from build123d import *

# Parameters (mm, degrees)
CUT_EXTRUDE_1_REACH              = 10
HOLE_WIZARD_M41_AT_2_COUNT       = 2
HOLE_WIZARD_M41_AT_2_PITCH       = 24.04163056
HOLE_WIZARD_M41_AT_3_COUNT       = 2
HOLE_WIZARD_M41_AT_3_PITCH       = 34
HOLE_WIZARD_M41_AT_4_COUNT       = 2
HOLE_WIZARD_M41_AT_4_PITCH       = 24.04163056
HOLE_WIZARD_8_2_8_2_1_AT_2_COUNT = 2
HOLE_WIZARD_8_2_8_2_1_AT_2_PITCH = 29.69848481
HOLE_WIZARD_8_2_8_2_1_AT_3_COUNT = 2
HOLE_WIZARD_8_2_8_2_1_AT_3_PITCH = 42
HOLE_WIZARD_8_2_8_2_1_AT_4_COUNT = 2
HOLE_WIZARD_8_2_8_2_1_AT_4_PITCH = 29.69848481


with BuildPart() as part:
    # Эскиз1 → Повернуть1 (revolve)
    with BuildSketch(Plane.XY):
        with BuildLine():
            Line((7.5, 11), (0.5, 11))
            Line((0.5, 11), (0, 11.5))
            Line((0, 11.5), (0, 25.5))
            Line((0, 25.5), (0.5, 26))
            Line((0.5, 26), (5.5, 26))
            Line((5.5, 26), (6, 25.5))
            Line((6, 25.5), (6, 13.35))
            ThreePointArc((6, 13.35), (6.117157288, 13.067157288), (6.4, 12.95))
            Line((6.4, 12.95), (7.5, 12.95))
            Line((7.5, 12.95), (8, 12.45))
            Line((8, 12.45), (8, 11.5))
            Line((8, 11.5), (7.5, 11))
        make_face()
    revolve(axis=Axis((0, 0, 0), (1, 0, 0)))

    # Эскиз2 → Вырез-Вытянуть1 (cut, up to next)
    with BuildSketch(Plane.ZY, mode=Mode.PRIVATE) as cut_extrude_1_sk1:
        with BuildLine():
            Line((-15.329709717, 21), (15.329709717, 21))
            ThreePointArc((15.329709717, 21), (0, 26), (-15.329709717, 21))
        make_face()
    cut_extrude_1_tool1 = extrude(cut_extrude_1_sk1.sketch, amount=-CUT_EXTRUDE_1_REACH, mode=Mode.PRIVATE) & part.part
    add(cut_extrude_1_tool1.solids().sort_by_distance((0, 23.017458, 0))[0], mode=Mode.SUBTRACT)
    # Эскиз2 → Вырез-Вытянуть1 (cut, up to next)
    with BuildSketch(Plane.ZY, mode=Mode.PRIVATE) as cut_extrude_1_sk2:
        with BuildLine():
            Line((21, 15.329709717), (21, -15.329709717))
            ThreePointArc((21, -15.329709717), (26, 0), (21, 15.329709717))
        make_face()
    cut_extrude_1_tool2 = extrude(cut_extrude_1_sk2.sketch, amount=-CUT_EXTRUDE_1_REACH, mode=Mode.PRIVATE) & part.part
    add(cut_extrude_1_tool2.solids().sort_by_distance((0, 0, 23.017458))[0], mode=Mode.SUBTRACT)
    # Эскиз2 → Вырез-Вытянуть1 (cut, up to next)
    with BuildSketch(Plane.ZY, mode=Mode.PRIVATE) as cut_extrude_1_sk3:
        with BuildLine():
            Line((15.329709717, -21), (-15.329709717, -21))
            ThreePointArc((-15.329709717, -21), (0, -26), (15.329709717, -21))
        make_face()
    cut_extrude_1_tool3 = extrude(cut_extrude_1_sk3.sketch, amount=-CUT_EXTRUDE_1_REACH, mode=Mode.PRIVATE) & part.part
    add(cut_extrude_1_tool3.solids().sort_by_distance((0, -23.017458, 0))[0], mode=Mode.SUBTRACT)
    # Эскиз2 → Вырез-Вытянуть1 (cut, up to next)
    with BuildSketch(Plane.ZY, mode=Mode.PRIVATE) as cut_extrude_1_sk4:
        with BuildLine():
            Line((-21, -15.329709717), (-21, 15.329709717))
            ThreePointArc((-21, 15.329709717), (-26, 0), (-21, -15.329709717))
        make_face()
    cut_extrude_1_tool4 = extrude(cut_extrude_1_sk4.sketch, amount=-CUT_EXTRUDE_1_REACH, mode=Mode.PRIVATE) & part.part
    add(cut_extrude_1_tool4.solids().sort_by_distance((0, 0, -23.017458))[0], mode=Mode.SUBTRACT)

    # Эскиз4 → Цековка для винта с внутренним шестигранником M41 (revolve, cut)
    with BuildSketch(Plane(origin=(0, 15.974774553, 5.814342437), x_dir=(0, 0, 1), z_dir=(0, 1, 0))):
        Polygon((0, 0), (0, 6), (2.4, 6), (2.25, 5.85), (2.25, 4.2), (3.7, 4.2), (3.7, 0.15), (3.85, 0), align=None)
    hole_wizard_m41 = revolve(axis=Axis((-6.35, 15.974774553, 5.814342437), (1, 0, 0)), mode=Mode.SUBTRACT)

    # Цековка для винта с внутренним шестигранником M41 at 2: Цековка для винта с внутренним шестигранником M41 ×2
    with Locations(*[Vector(0, -0.422618262, -0.906307787) * (i * HOLE_WIZARD_M41_AT_2_PITCH) for i in range(1, HOLE_WIZARD_M41_AT_2_COUNT)]):
        add(hole_wizard_m41, mode=Mode.SUBTRACT)

    # Цековка для винта с внутренним шестигранником M41 at 3: Цековка для винта с внутренним шестигранником M41 ×2
    with Locations(*[Vector(0, -0.939692621, -0.342020143) * (i * HOLE_WIZARD_M41_AT_3_PITCH) for i in range(1, HOLE_WIZARD_M41_AT_3_COUNT)]):
        add(hole_wizard_m41, mode=Mode.SUBTRACT)

    # Цековка для винта с внутренним шестигранником M41 at 4: Цековка для винта с внутренним шестигранником M41 ×2
    with Locations(*[Vector(0, -0.906307787, 0.422618262) * (i * HOLE_WIZARD_M41_AT_4_PITCH) for i in range(1, HOLE_WIZARD_M41_AT_4_COUNT)]):
        add(hole_wizard_m41, mode=Mode.SUBTRACT)

    # Эскиз6 → Диаметр отверстия Ø8.2 (8.2)1 (revolve, cut)
    with BuildSketch(Plane(origin=(0, 14.849242405, -14.849242405), x_dir=(0, 0, 1), z_dir=(0, 1, 0))):
        Polygon((0, 0), (0, 6), (4.25, 6), (4.1, 5.85), (4.1, 0.15), (4.25, 0), align=None)
    hole_wizard_8_2_8_2_1 = revolve(axis=Axis((-6.35, 14.849242405, -14.849242405), (1, 0, 0)), mode=Mode.SUBTRACT)

    # Диаметр отверстия Ø8.2 (8.2)1 at 2: Диаметр отверстия Ø8.2 (8.2)1 ×2
    with Locations(*[(0, 0, i * HOLE_WIZARD_8_2_8_2_1_AT_2_PITCH) for i in range(1, HOLE_WIZARD_8_2_8_2_1_AT_2_COUNT)]):
        add(hole_wizard_8_2_8_2_1, mode=Mode.SUBTRACT)

    # Диаметр отверстия Ø8.2 (8.2)1 at 3: Диаметр отверстия Ø8.2 (8.2)1 ×2
    with Locations(*[Vector(0, -0.707106781, 0.707106781) * (i * HOLE_WIZARD_8_2_8_2_1_AT_3_PITCH) for i in range(1, HOLE_WIZARD_8_2_8_2_1_AT_3_COUNT)]):
        add(hole_wizard_8_2_8_2_1, mode=Mode.SUBTRACT)

    # Диаметр отверстия Ø8.2 (8.2)1 at 4: Диаметр отверстия Ø8.2 (8.2)1 ×2
    with Locations(*[(0, -i * HOLE_WIZARD_8_2_8_2_1_AT_4_PITCH, 0) for i in range(1, HOLE_WIZARD_8_2_8_2_1_AT_4_COUNT)]):
        add(hole_wizard_8_2_8_2_1, mode=Mode.SUBTRACT)


solid = part.part
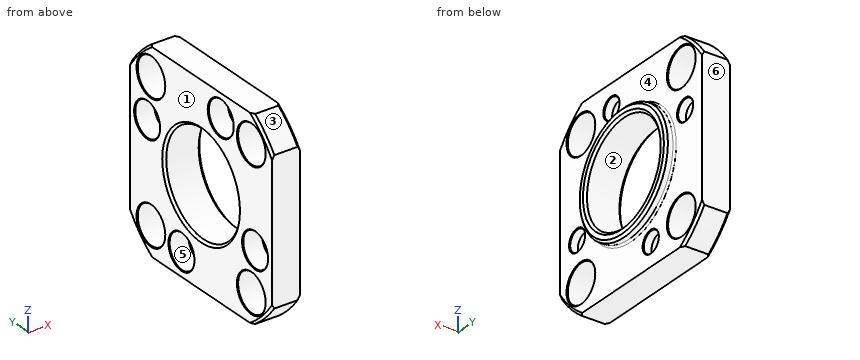
Geometry check sheet. Reference: the model listing, model coordinates, mm. Face numbers are marked on the shaded views. A direction names the side the tool comes from. Round coordinates to 2 decimals unless told otherwise and drop trailing zeros. Write each loop counter-clockwise with the first axis right and the second up, starting at its lowest first coordinate (ties: lowest second). Pieces come first, ordered by that corner, then holes. Notation, with made-up numbers: (3, 86) -> (9, 86) arc R10 ccw to (9, 93) -> close; hole circle Ø6 at (-7, 26). An arc over 180 degrees is marked (long way). One line per item, written item: value. Start each with the question number.
(1) Access from +Z, -Z, +X, -X, +Y, -Y to the whole of each face (thin tool, end or side, straight path). Record for the marked faces 4, 5 and 6.
(2) Go/stop test with flat-tipped pins: pin 1 Ø6 at (y, z) = (-15.97, -5.81) entering from -X; pin 2 Ø6 at (y, z) = (-5.81, 15.97) entering from +X. Record where each tip stops, or that it passes through.
(3) Cross-section at C-C, the plane x = 1.5. Give the number of separate pieces and of enclosed holes in the cut face, and give its area (3 significant figures).
(4) Draft check along Y on the marked faces 1, 2 and 3. Enter one of: +Y half, -Y half, draft (parallel to the pull), parting line (faces both ways), or undercut.
(5) Cross-section at A-A, the plane z = 0. Record the cut outline in (x, y), and give its area (3 significant figures).
(6) Scan lines: line 1 (Z direction, x = 4.75, y = 0.5); line 2 (Z direction, x = 5.25, y = -5.5); line 3 (Z direction, x = 2, y = 6). Record each from-to range of solid material in increasing order. Write a range as [from, to].
Answer:
1. face 4: +X
1. face 5: -X
1. face 6: +Z, -Z, +X, -X, +Y
2. pin 1: x = 4.2
2. pin 2: x = 6
3. separate pieces: 1
3. enclosed holes: 9
3. area: 943 mm²
4. face 1: draft
4. face 2: undercut
4. face 3: -Y half
5. outline: (0, -21) -> (6, -21) -> (6, -13.35) arc R0.4 cw to (6.4, -12.95) -> (7.5, -12.95) -> (8, -12.45) -> (8, -11.5) -> (7.5, -11) -> (0.5, -11) -> (0, -11.5) -> close; (0, 11.5) -> (0.5, 11) -> (7.5, 11) -> (8, 11.5) -> (8, 12.45) -> (7.5, 12.95) -> (6.4, 12.95) arc R0.4 cw to (6, 13.35) -> (6, 21) -> (0, 21) -> close
5. area: 127 mm²
6. line 1: [-21, -10.99], [10.99, 21]
6. line 2: [-21, -9.53], [9.53, 13.75], [18.2, 21]
6. line 3: [-21, -19.67], [-12.28, -9.22], [9.22, 21]
